For this review, take the finished solid that the model builds, in its own axes (mm). A direction names the side the tool comes from. Give positions to 0.01 mm unless a question says otherwise; leave off trailing zeros. Loops run counter-clockwise (first coordinate to the right, second up) from the corner with the lowest first, then second, coordinate; pieces in that order, holes last. Notation, with made-up numbers: (-2, 64.5) - (44, 64.5) arc R17 ccw to (44, 88.5) - close; hole circle Ø7 at (62, 67.5). An arc over 180 degrees is marked (long way). Put each result on its own line as item: value. Start each with the question number.
from build123d import *

# Parameters (mm, degrees)
F0_W     = 23
F0_H     = 15.370602
F1_DEPTH = 39
F2_DEPTH = 2
F3_T     = -2.5


with BuildPart() as f1:
    # F0 (on Top) → F1 (new body)
    with BuildSketch(Plane.XY):
        with Locations((0, -17.314699)):
            Rectangle(F0_W, F0_H)
    extrude(amount=F1_DEPTH)

    # F0 (on Top) → F2 (join)
    with BuildSketch(Plane.XY):
        Polygon((25, 25), (-25, 25), (-25, -25), (-11.5, -25), (-11.5, -9.629398), (11.5, -9.629398), (11.5, -25), (25, -25), align=None)
    extrude(amount=F2_DEPTH)

    # F3
    f3_openings = [f1.faces().sort_by_distance(p)[0] for p in [
        (0, -25, 18.449527),
    ]]
    offset(amount=F3_T, openings=f3_openings)


solid = f1.part
1) Take a section at A-A on x = -8. State the section outline as (y, z) points, and give its area (3 significant figures).
2) Machinability: for faces 1 (the flat face through (0, -9.629, 20)), 2 (the flat face through (-11.5, -17, 20)), 3 (the flat face through (0, -18, 36.5)), which of the approach directions +Z, -Z, +X, -X, +Y, -Y give a long, thin tool a straight path to every point of the face, cutting with its end or side? Answer none if there is none.
3) Insertion check: P1, Ø4, axis at y = -17, z = 14, coming from the +X side; P2, Ø2, axis at x = -4.5, z = 12.5, coming from the -Y side; P3, Ø4.5, axis at y = -14.5, z = 28, coming from the -X side. Each pin has a flat end and moves straight along its axis. Give the tip position at first contact, or say it passes through.
4) Take a section at C-C on y = 0. State the section outline as (x, z) points.
5) Mouldability with a two-part tool opening along X and no side actions: class faces 4 (the flat face through (9, -19, 19)), 5 (the flat face through (0, 0, 0)), 6 (the flat face through (-25, 0, 1)), 7 (the flat face through (-9, -19, 19)) as released by +X, released by -X, zero draft, split by the parting line, or undercut.
6) Take a section at B-B on z = 28.5. State the section outline as (x, y) points.
7) Wall thickness on probe 1 along X at (y, z) = (-22, 16); probe 2 along Z at (x, y) = (3, -18.5); probe 3 along Z at (x, y) = (-23, -4): over which ranges is each line inside the solid? List them lowest first.
Answers follow:
1. outline: (-25, 0) - (25, 0) - (25, 2) - (-9.63, 2) - (-9.63, 39) - (-25, 39) - (-25, 36.5) - (-12.13, 36.5) - (-12.13, 2.5) - (-25, 2.5) - close
1. area: 231 mm2
2. face 1: +Z, +X, -X, +Y
2. face 2: +Z, -X, +Y, -Y
2. face 3: -Y
3. P1: x = 11.5
3. P2: y = -12.13
3. P3: x = -11.5
4. outline: (-25, 0) - (25, 0) - (25, 2) - (-25, 2) - close
5. face 4: undercut
5. face 5: zero draft
5. face 6: released by -X
5. face 7: undercut
6. outline: (-11.5, -25) - (-9, -25) - (-9, -12.13) - (9, -12.13) - (9, -25) - (11.5, -25) - (11.5, -9.63) - (-11.5, -9.63) - close
7. probe 1: -11.5 to -9, 9 to 11.5
7. probe 2: 0 to 2.5, 36.5 to 39
7. probe 3: 0 to 2
